```python
from build123d import *

# Parameters (mm, degrees)
BOSS_EXTRUDE1_DEPTH = 1.5875
CUT_EXTRUDE1_DEPTH  = 10
CUT_EXTRUDE2_DEPTH  = 399.337162784


with BuildPart() as part:
    # Sketch1 → Boss-Extrude1 (new, symmetric)
    with BuildSketch(Plane.XY):
        with BuildLine():
            Line((118.523395286, 71.943678131), (118.634293919, 75.116740767))
            ThreePointArc((118.634293919, 75.116740767), (103.883786228, 214.067962894), (128.160173541, 351.674927204))
            ThreePointArc((128.160173541, 351.674927204), (120.284402828, 355.375683964), (112.284762731, 358.800464724))
            Line((112.284762731, 358.800464724), (103.942723114, 335.880899242))
            ThreePointArc((103.942723114, 335.880899242), (91.734409036, 330.188068894), (86.041578688, 342.396382972))
            Line((86.041578688, 342.396382972), (94.383618305, 365.315948454))
            ThreePointArc((94.383618305, 365.315948454), (82.568877465, 368.795382466), (70.597294753, 371.689474641))
            Line((70.597294753, 371.689474641), (66.36193024, 347.669528881))
            ThreePointArc((66.36193024, 347.669528881), (55.3276375, 339.943233926), (47.601342545, 350.977526666))
            Line((47.601342545, 350.977526666), (51.836707058, 374.997472425))
            ThreePointArc((51.836707058, 374.997472425), (39.597261303, 376.3724378), (27.305, 377.14371869))
            Line((27.305, 377.14371869), (27.305, 352.825))
            ThreePointArc((27.305, 352.825), (17.78, 343.3), (8.255, 352.825))
            Line((8.255, 352.825), (8.255, 377.14371869))
            ThreePointArc((8.255, 377.14371869), (-4.037261303, 376.3724378), (-16.276707058, 374.997472425))
            Line((-16.276707058, 374.997472425), (-12.041342545, 350.977526666))
            ThreePointArc((-12.041342545, 350.977526666), (-19.7676375, 339.943233926), (-30.80193024, 347.669528881))
            Line((-30.80193024, 347.669528881), (-35.037294753, 371.689474641))
            ThreePointArc((-35.037294753, 371.689474641), (-47.008877465, 368.795382466), (-58.823618305, 365.315948454))
            Line((-58.823618305, 365.315948454), (-50.481578688, 342.396382972))
            ThreePointArc((-50.481578688, 342.396382972), (-56.174409036, 330.188068894), (-68.382723114, 335.880899242))
            Line((-68.382723114, 335.880899242), (-76.724762731, 358.800464724))
            ThreePointArc((-76.724762731, 358.800464724), (-88.8119245, 353.496726812), (-100.602714669, 347.563230147))
            ThreePointArc((-100.602714669, 347.563230147), (-76.713636703, 301.658133404), (-41.846325708, 263.418931306))
            ThreePointArc((-41.846325708, 263.418931306), (-13.109519742, 151.040608787), (-109.894880363, 87.108728174))
            Line((-109.894880363, 87.108728174), (-110.145579114, 79.935665538))
            Line((-110.145579114, 79.935665538), (-100.151681047, 79.586378505))
            Line((-100.151681047, 79.586378505), (-100.040782415, 82.759441142))
            Line((-100.040782415, 82.759441142), (-55.365911398, 81.198053081))
            Line((-55.365911398, 81.198053081), (-55.476810031, 78.024990444))
            Line((-55.476810031, 78.024990444), (-45.482911964, 77.675703412))
            Line((-45.482911964, 77.675703412), (-45.372013331, 80.848766048))
            Line((-45.372013331, 80.848766048), (-0.697142315, 79.287377987))
            Line((-0.697142315, 79.287377987), (-0.808040947, 76.114315351))
            Line((-0.808040947, 76.114315351), (9.185857119, 75.765028318))
            Line((9.185857119, 75.765028318), (9.296755752, 78.938090955))
            Line((9.296755752, 78.938090955), (53.971626769, 77.376702893))
            Line((53.971626769, 77.376702893), (53.860728136, 74.203640257))
            Line((53.860728136, 74.203640257), (63.854626203, 73.854353225))
            Line((63.854626203, 73.854353225), (63.965524835, 77.027415861))
            Line((63.965524835, 77.027415861), (72.0752213, 76.74398173))
            Line((72.0752213, 76.74398173), (73.821656463, 126.713472064))
            ThreePointArc((73.821656463, 126.713472064), (75.463637097, 128.244554066), (76.994719099, 126.602573431))
            Line((76.994719099, 126.602573431), (75.248283936, 76.633083097))
            Line((75.248283936, 76.633083097), (108.640395852, 75.4660278))
            Line((108.640395852, 75.4660278), (108.529497219, 72.292965164))
            Line((108.529497219, 72.292965164), (118.523395286, 71.943678131))
        make_face()
        with BuildLine():
            Line((79.934179532, 301.606688232), (80.807397113, 326.591433399))
            ThreePointArc((80.807397113, 326.591433399), (82.449377747, 328.122515401), (83.980459749, 326.480534766))
            Line((83.980459749, 326.480534766), (83.107242168, 301.4957896))
            ThreePointArc((83.107242168, 301.4957896), (81.465261533, 299.964707598), (79.934179532, 301.606688232))
        make_face(mode=Mode.SUBTRACT)
        with BuildLine():
            ThreePointArc((79.614371843, 201.556808932), (77.972391208, 200.02572693), (76.441309207, 201.667707565))
            Line((76.441309207, 201.667707565), (77.314526788, 226.652452732))
            ThreePointArc((77.314526788, 226.652452732), (78.956507422, 228.183534733), (80.487589424, 226.541554099))
            Line((80.487589424, 226.541554099), (79.614371843, 201.556808932))
        make_face(mode=Mode.SUBTRACT)
    extrude(amount=BOSS_EXTRUDE1_DEPTH, both=True)

    # Sketch2 → Cut-Extrude1 (cut)
    with BuildSketch(Plane.XY.offset(1.5875)):
        with BuildLine():
            ThreePointArc((59.060719004, 274.255221739), (16.218243133, 313.208722852), (-4.20589422, 259.026552342))
            ThreePointArc((-4.20589422, 259.026552342), (17.803012445, 201.122949157), (9.309397428, 139.762719868))
            ThreePointArc((9.309397428, 139.762719868), (29.062919552, 105.536460681), (57.283668785, 133.199211213))
            ThreePointArc((57.283668785, 133.199211213), (53.631087043, 203.784426197), (59.060719004, 274.255221739))
        make_face()
    extrude(amount=-CUT_EXTRUDE1_DEPTH, mode=Mode.SUBTRACT)

    # Sketch3 → Cut-Extrude2 (cut, through all)
    with BuildSketch(Plane.XY.offset(1.5875)):
        with BuildLine():
            Line((-87.375537588, 354.172706758), (-83.117396192, 345.124600224))
            ThreePointArc((-83.117396192, 345.124600224), (-83.877803157, 343.012233365), (-85.990170016, 343.772640331))
            Line((-85.990170016, 343.772640331), (-90.248311413, 352.820746865))
            ThreePointArc((-90.248311413, 352.820746865), (-89.487904447, 354.933113724), (-87.375537588, 354.172706758))
        make_face()
        with BuildLine():
            Line((-45.475470216, 369.2062577), (-42.887279765, 359.546999437))
            ThreePointArc((-42.887279765, 359.546999437), (-44.00981178, 357.602716954), (-45.954094263, 358.725248969))
            Line((-45.954094263, 358.725248969), (-48.542284715, 368.384507232))
            ThreePointArc((-48.542284715, 368.384507232), (-47.419752699, 370.328789715), (-45.475470216, 369.2062577))
        make_face()
        with BuildLine():
            Line((-2.45580222, 376.510797541), (-1.584244793, 366.548850561))
            ThreePointArc((-1.584244793, 366.548850561), (-3.027344134, 364.829031736), (-4.747162959, 366.272131077))
            Line((-4.747162959, 366.272131077), (-5.618720387, 376.234078058))
            ThreePointArc((-5.618720387, 376.234078058), (-4.175621045, 377.953896883), (-2.45580222, 376.510797541))
        make_face()
        with BuildLine():
            Line((41.178720387, 376.234078058), (40.307162959, 366.272131077))
            ThreePointArc((40.307162959, 366.272131077), (38.587344134, 364.829031736), (37.144244793, 366.548850561))
            Line((37.144244793, 366.548850561), (38.01580222, 376.510797541))
            ThreePointArc((38.01580222, 376.510797541), (39.735621045, 377.953896883), (41.178720387, 376.234078058))
        make_face()
        with BuildLine():
            Line((84.102284715, 368.384507232), (81.514094263, 358.725248969))
            ThreePointArc((81.514094263, 358.725248969), (79.56981178, 357.602716954), (78.447279765, 359.546999437))
            Line((78.447279765, 359.546999437), (81.035470216, 369.2062577))
            ThreePointArc((81.035470216, 369.2062577), (82.979752699, 370.328789715), (84.102284715, 368.384507232))
        make_face()
        with BuildLine():
            Line((121.732705627, 354.725626081), (117.637852823, 345.60245884))
            ThreePointArc((117.637852823, 345.60245884), (115.539492141, 344.804213923), (114.741247224, 346.902574605))
            Line((114.741247224, 346.902574605), (118.836100028, 356.025741846))
            ThreePointArc((118.836100028, 356.025741846), (120.934460711, 356.823986763), (121.732705627, 354.725626081))
        make_face()
    extrude(amount=-CUT_EXTRUDE2_DEPTH, mode=Mode.SUBTRACT)


solid = part.part
```
Model file for the job. Use its own axes, mm. A direction names the side the tool comes from. Coordinates: 2 decimals unless noted, no trailing zeros. Loops run counter-clockwise (first coordinate to the right, second up) from the corner with the lowest first, then second, coordinate; pieces in that order, holes last. Notation, with made-up numbers: (82.25, 64) - (108.25, 64) arc R12 ccw to (108.25, 82) - close; hole circle Ø7 at (-2, 52.5). An arc over 180 degrees is marked (long way). Answer as a JSON object with one key per item and string values. Group by question number.
(1) Cut at D-D (y = 317.5). Give the cut face in (x, z), then the cut area to 3 significant figures.
(2) Cut at C-C (z = -0.15). State how many separate pieces and enclosed holes the cut face has, then the cut area to 3 significant figures.
(3) Cut at A-A (y = 92). Give the cut face in (x, z), then the cut area to 3 significant figures.
(4) Cut at B-B (y = 216). Give the cut face in (x, z).
(5) Flat gauge pins, fed straight in: pin 1 (1 mm diameter, centred on x = 11, z = 0, fed in from -Y); pin 2 (1 mm diameter, centred on y = 198.5, z = -1, fed in from +X); pin 3 (1.6 mm diameter, centred on y = 362.5, z = -0.5, fed in from -X). Where does each tip first touch, or does it go through?
(6) Two-plate mould, pull along X, no slides. Class faces 1 (the face through (-55.98, 330.26, 0.02)), 2 (the face through (7, 227, -1.588)), 3 (the face through (17.15, 313.42, 0.02)), 4 (the face through (103.82, 212.11, 0.02)): released by +X, released by -X, zero draft, split by the parting line, or undercut.
(7) Probe line 1 along X through (y, z) = (331.5, 0.15); line 2 along X through (y, z) = (206, -0.2); line 3 along X through (y, z) = (260, 0). List the from-to ranges inside material, lowest first.
(8) Tool access for faces 5 (the face through (108.17, 347.5, 0.02)), 6 (the face through (-77.129, 302.255, 0.022)), 7 (the face through (17.7, 202, 0)): list every direction of +Z, -Z, +X, -X, +Y, -Y with a clear straight run to the whole face (end or side of a thin tool).
Geometry says:
{
 "1": {"outline": "(-86.71, -1.59) - (80.49, -1.59) - (80.49, 1.59) - (-86.71, 1.59) - close; (83.67, -1.59) - (118.36, -1.59) - (118.36, 1.59) - (83.67, 1.59) - close", "area": "641 mm^2"},
 "2": {"separate pieces": "1", "enclosed holes": "3", "area": "32,500 mm^2"},
 "3": {"outline": "(-75.32, -1.59) - (72.61, -1.59) - (72.61, 1.59) - (-75.32, 1.59) - close; (75.79, -1.59) - (114.71, -1.59) - (114.71, 1.59) - (75.79, 1.59) - close", "area": "593 mm^2"},
 "4": {"outline": "(-10.68, -1.59) - (15.2, -1.59) - (15.2, 1.59) - (-10.68, 1.59) - close; (53.92, -1.59) - (76.94, -1.59) - (76.94, 1.59) - (53.92, 1.59) - close; (80.12, -1.59) - (103.95, -1.59) - (103.95, 1.59) - (80.12, 1.59) - close"},
 "5": {"pin 1": "stops at y = 78.86", "pin 2": "stops at x = 103.59", "pin 3": "stops at x = -58.09"},
 "6": {"face 1": "undercut", "face 2": "zero draft", "face 3": "undercut", "face 4": "released by +X"},
 "7": {"line 1": "x = -93.93 to -65.12, -53.74 to 89.3, 100.68 to 122.06", "line 2": "x = -8.21 to 17.15, 53.66 to 76.59, 79.77 to 103.67", "line 3": "x = -38.01 to -4.87, 57.22 to 107.59"},
 "8": {"face 5": "+Z, -Z, +Y", "face 6": "+Z, -Z, -X", "face 7": "+Z, -Z"}
}
